from build123d import *

# Parameters (mm, degrees)
F0_W     = 35.83182
F0_H     = 3.02196
F1_DEPTH = 26
F2_R     = 2.558205
F3_DEPTH = 6
F5_DEPTH = 3


with BuildPart() as f1:
    # F0 (on Front) → F1 (new body)
    with BuildSketch(Plane.XZ):
        with Locations((17.91591, 1.51098)):
            Rectangle(F0_W, F0_H)
    extrude(amount=F1_DEPTH)

    # F2 (on Front) → F3 (join)
    with BuildSketch(Plane.XZ):
        with BuildLine():
            Line((0, 2.911769), (35.83182, 2.911769))
            Line((35.83182, 2.911769), (21.992884, 25.98811))
            ThreePointArc((21.992884, 25.98811), (17.91591, 28.297043), (13.838936, 25.98811))
            Line((13.838936, 25.98811), (0, 2.911769))
        make_face()
        with Locations((17.91591, 23.543139)):
            Circle(F2_R, mode=Mode.SUBTRACT)
    extrude(amount=F3_DEPTH)

    # F4 (on face) → F5 (join)
    with BuildSketch(Plane.XZ.offset(26)):
        Polygon((0, 3.02196), (0, 0), (11.269107, 0), (11.269107, 7.273588), (7.463317, 7.273588), align=None)
        Polygon((24.689507, 0), (35.83182, 0), (35.83182, 3.02196), (28.895905, 7.273588), (24.689507, 7.273588), align=None)
    extrude(amount=F5_DEPTH)


solid = f1.part
Read the model definition and answer for the solid it produces. Units are mm, in the model's axes. A direction names the side the tool comes from. Round coordinates to 2 decimals unless told otherwise and drop trailing zeros. Loops run counter-clockwise (first coordinate to the right, second up) from the corner with the lowest first, then second, coordinate; pieces in that order, holes last.
Q1. Section A-A on z = 3.5 is taken. Write down the section's boundary in (x, y), and give its area (3 significant figures).
Q2. Determine the mould class of faces 1 (the face through (18, -16, 3.022)), 2 (the face through (32.41, -27.48, 5.12)), 3 (the face through (15.886, -2.958, 21.987)) for opening direction X: released by +X, released by -X, zero draft, split by the parting line, or undercut.
Q3. Consider probe 1 along Y at (x, z) = (10.5, 6.5); probe 2 along Y at (x, z) = (15, 3.75); probe 3 along Z at (x, y) = (26, -9.25). Determine where each line is inside the solid, lowest interval first.
Q4. Section B-B on x = 16.5 is taken. Write down the section's boundary in (y, z).
Q5. Each of these flat-tipped pins is pushed along its axis until it touches: pin 1 (1.5 mm diameter, centred on x = 4, z = 10.5, fed in from -Y); pin 2 (1.5 mm diameter, centred on x = 15, y = -7, fed in from +Z); pin 3 (0.9 mm diameter, centred on x = 9, y = -27, fed in from +Z); pin 4 (1.3 mm diameter, centred on x = 5.5, z = 6, fed in from +Y). Where does it stop, or does it pass through?
Q6. Section C-C on x = 6.5 is taken. Write down the section's boundary in (y, z).
Q7. Which of the six approach directions +Z, -Z, +X, -X, +Y, -Y give full straight-line access (tool end or side, diameter ignored) to faces 4 (the face through (24.69, -27, 4)), 5 (the face through (29, -26, 5)), 6 (the face through (3.784, -27.479, 5.178))?
Q8. Section D-D on z = 25.5 is taken. Write down the section's boundary in (x, y), and give its area (3 significant figures).
Output:
1. outline: (0.35, -6) - (35.48, -6) - (35.48, 0) - (0.35, 0) - close; (0.84, -29) - (11.27, -29) - (11.27, -26) - (0.84, -26) - close; (24.69, -29) - (35.05, -29) - (35.05, -26) - (24.69, -26) - close
1. area: 273 mm2
2. face 1: zero draft
2. face 2: released by +X
2. face 3: undercut
3. probe 1: y = -29 to -26, -6 to 0
3. probe 2: y = -6 to 0
3. probe 3: z = 0 to 3.02
4. outline: (-26, 0) - (0, 0) - (0, 21.41) - (-6, 21.41) - (-6, 3.02) - (-26, 3.02) - close; (-6, 25.67) - (0, 25.67) - (0, 28.08) - (-6, 28.08) - close
5. pin 1: stops at y = -6
5. pin 2: stops at z = 3.02
5. pin 3: stops at z = 7.27
5. pin 4: stops at y = 0
6. outline: (-29, 0) - (0, 0) - (0, 13.75) - (-6, 13.75) - (-6, 3.02) - (-26, 3.02) - (-26, 6.72) - (-29, 6.72) - close
7. face 4: +Z, -Z, -Y
7. face 5: +Z, +X, -X
7. face 6: +Z, -X, -Y
8. outline: (13.55, -6) - (16.27, -6) - (16.27, 0) - (13.55, 0) - close; (19.56, -6) - (22.29, -6) - (22.29, 0) - (19.56, 0) - close
8. area: 32.7 mm2
